Source: CAD feature listing. Evaluate the final solid. Frame: model axes, mm. A direction names the side the tool comes from. Coordinates: 2 decimals unless noted, no trailing zeros. Order: outer loops, then holes, each group sorted by start corner. A loop starts at its lowest first (then second) coordinate and runs counter-clockwise, first axis right, second up. Notation, with made-up numbers: (-34, -16.75) - (-8, -16.75) arc R21 cw to (-8, 1.25) - close; hole circle Ø11 at (-6.75, 30). An arc over 180 degrees is marked (long way). One line per question, with ' | ' between items. Start each with the question number.
(1) Draft query along Y for faces 4 (the flat face through (22, 0, 9.525)), 5 (the cylindrical face through (34.109, 14.664, -6.08)), 6 (the flat face through (3.175, 10, 14)), 7 (the flat face through (18, 12.7, 11)). Return one class per face: +Y half, -Y half, draft (parallel to the pull), parting line (faces both ways), or undercut.
(2) Section B-B (y = -9.5). Return the cut outline in (x, z) (1 decimal).
(3) Section D-D (z = -5). Return the cut outline in (x, y) (3 decimals).
(4) Section A-A (z = 4.5). Return the cut outline in (x, y) (3 decimals), then the cut area to 3 significant figures.
(5) Section C-C (x = 10). Count the separate pieces of the cut face and the enclosed holes in it, then the cut area to 3 significant figures.
(6) Line query: line 1 along Z through (x, y) = (21, 0) (1 decimal); line 2 along Z through (x, y) = (18, 0) (1 decimal); line 3 along X through (y, z) = (-5.5, 12.7). Output: solid intervals per line, ascending.
(7) Access query for faces 1 (the flat face through (3.175, 15.4, 4.8)), 2 (the flat face through (18, 0, 9.525)), 3 (the cylindrical face through (18.71, -8, 14.04)). Directions: +Z, -Z, +X, -X, +Y, -Y. A direction counts if a zero-diameter tool reaches every point of the face in a straight line with its end or side. Return the directions, or none.
(8) Contact query for flat-ended pins moving along their axis: P1, Ø5, axis at x = 18.5, z = 9, coming from the +Y side; P2, Ø5, axis at x = 28, z = 4.5, coming from the -Y side; P3, Ø0.8, axis at x = 35, z = 8.5, coming from the +Y side. Output: stop coordinate, or through.
from build123d import *

# Parameters (mm, degrees)
F0_R      = 15.875
F1_DEPTH  = 35.71875
F2_W      = 29.36875
F2_H      = 3.175
F4_W      = 29.36875
F4_H      = 25.4
F5_DEPTH  = 15.875
F6_W      = 29.36875
F6_H      = 12.7
F7_DEPTH  = 15.875
F8_R      = 7.9375
F9_DEPTH  = 35.71975
F10_W     = 1.5875
F10_H     = 6.35
F10_W_2   = 3.175
F11_DEPTH = 6.35
F12_R     = 1.5875
F13_DEPTH = 12.7
F15_W     = 9.525
F15_H     = 6.0325
F16_DEPTH = 1.5875
F17_W     = 9.525
F17_H     = 6.0325
F18_DEPTH = 1.5875
F22_R     = 1.2446
F23_DEPTH = 13.97
F27_R     = 1.2446
F28_DEPTH = 13.97


with BuildPart() as f1:
    # F0 (on Right) → F1 (new body)
    with BuildSketch(Plane.YZ):
        Circle(F0_R)
    extrude(amount=F1_DEPTH)

    # F2 (on Front) → F3 (revolve, cut)
    with BuildSketch(Plane.XZ):
        with Locations((17.859375, 14.2875)):
            Rectangle(F2_W, F2_H)
    revolve(axis=Axis((19.161431, 0, 0), (1, 0, 0)), mode=Mode.SUBTRACT)

    # F4 (on Top) → F5 (join)
    with BuildSketch(Plane.XY):
        with Locations((17.859375, 0)):
            Rectangle(F4_W, F4_H)
    extrude(amount=F5_DEPTH)

    # F6 (on Front) → F7 (join)
    with BuildSketch(Plane.XZ):
        with Locations((17.859375, 0)):
            Rectangle(F6_W, F6_H)
    extrude(amount=-F7_DEPTH)

    # F8 (on face) → F9 (cut, through all)
    with BuildSketch(Plane.YZ.offset(35.71875)):
        Circle(F8_R)
    extrude(amount=-F9_DEPTH, mode=Mode.SUBTRACT)

    # F10 (on face) → F11 (cut)
    with BuildSketch(Plane.XY.offset(15.875)):
        with Locations((13.890625, 0)):
            Rectangle(F10_W, F10_H)
        with Locations((17.859375, 0)):
            Rectangle(F10_W_2, F10_H)
        with Locations((21.828125, 0)):
            Rectangle(F10_W, F10_H)
    extrude(amount=-F11_DEPTH, mode=Mode.SUBTRACT)

    # F12 (on face) → F13 (cut)
    with BuildSketch(Plane.XZ.offset(12.7)):
        with Locations((17.859375, 12.7)):
            Circle(F12_R)
    extrude(amount=-F13_DEPTH, mode=Mode.SUBTRACT)

    # F15 (on face) → F16 (cut)
    with BuildSketch(Plane.YZ.offset(35.71875)):
        with Locations((0, 8.09625)):
            Rectangle(F15_W, F15_H)
    extrude(amount=-F16_DEPTH, mode=Mode.SUBTRACT)

    # F17 (on face) → F18 (cut)
    with BuildSketch(Plane(origin=(0, 0, 0), x_dir=(0, -1, 0), z_dir=(-1, 0, 0))):
        with Locations((0, 8.09625)):
            Rectangle(F17_W, F17_H)
    extrude(amount=-F18_DEPTH, mode=Mode.SUBTRACT)

    # F22 (on face) → F23 (cut)
    with BuildSketch(Plane(origin=(32.393255, 0, -5.711805), x_dir=(0, 1, 0), z_dir=(0.984808, 0, -0.173648))):
        with Locations((2.54, 15.368172)):
            Circle(F22_R)
        with Locations((0, 15.368172)):
            Circle(F22_R)
        with Locations((-2.54, 15.368172)):
            Circle(F22_R)
    extrude(amount=-F23_DEPTH, mode=Mode.SUBTRACT)

    # F27 (on face) → F28 (cut)
    with BuildSketch(Plane(origin=(2.248443, 0, 0.396461), x_dir=(0, 1, 0), z_dir=(0.984808, 0, 0.173648))):
        with Locations((2.54, 9.165676)):
            Circle(F27_R)
        with Locations((-2.54, 9.165676)):
            Circle(F27_R)
        with Locations((0, 9.165676)):
            Circle(F27_R)
    extrude(amount=F28_DEPTH, mode=Mode.SUBTRACT)


solid = f1.part
Response values:
1) face 4: undercut | face 5: parting line | face 6: draft | face 7: +Y half
2) outline: (0, -12.7) - (3.2, -12.7) - (3.2, -8.4) - (32.5, -8.4) - (32.5, -12.7) - (35.7, -12.7) - (35.7, 12.7) - (32.5, 12.7) - (32.5, 15.9) - (3.2, 15.9) - (3.2, 12.7) - (0, 12.7) - close; hole circle Ø3.2 at (17.9, 12.7)
3) outline: (0, -15.067) - (3.175, -15.067) - (3.175, -11.674) - (32.544, -11.674) - (32.544, -15.067) - (35.719, -15.067) - (35.719, -6.165) - (0, -6.165) - close; (0, 6.165) - (35.719, 6.165) - (35.719, 15.067) - (32.544, 15.067) - (32.544, 15.875) - (3.175, 15.875) - (3.175, 15.067) - (0, 15.067) - close
4) outline: (0, -15.224) - (3.175, -15.224) - (3.175, -12.7) - (32.544, -12.7) - (32.544, -15.224) - (35.719, -15.224) - (35.719, -6.539) - (0, -6.539) - close; (0, 6.539) - (35.719, 6.539) - (35.719, 15.224) - (32.544, 15.224) - (32.544, 15.875) - (3.175, 15.875) - (3.175, 15.224) - (0, 15.224) - close | area: 565 mm²
5) separate pieces: 1 | enclosed holes: 4 | area: 488 mm²
6) line 1: z = -12.7 to -7.9, 7.9 to 15.9 | line 2: z = -12.7 to -7.9, 7.9 to 9.5 | line 3: x = 0 to 16.27, 19.45 to 35.72
7) face 1: +Z, -X, +Y | face 2: +Z | face 3: -Y
8) P1: stops at y = 12.7 | P2: stops at y = -12.7 | P3: stops at y = 13.65
